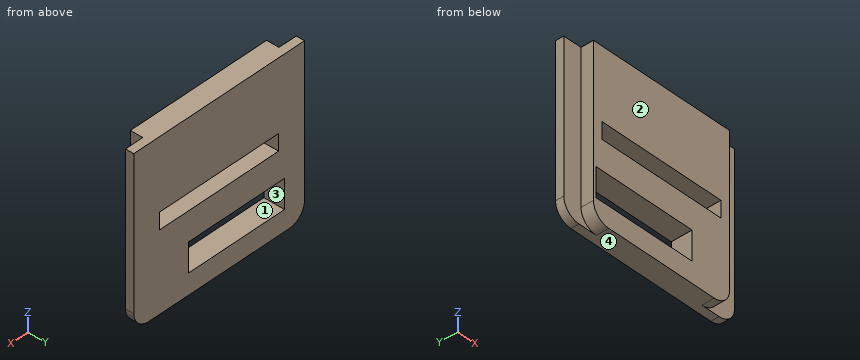
from build123d import *

# Parameters (mm, degrees)
F1_DEPTH = 1
F3_DEPTH = 1.5
F5_W     = 12.5
F5_H     = 3.5
F5_W_2   = 15.5
F5_H_2   = 2
F6_DEPTH = 2.5


with BuildPart() as f1:
    # F0 (on Front) → F1 (new body)
    with BuildSketch(Plane.XZ):
        with BuildLine():
            ThreePointArc((0, 2), (0.585786, 0.585786), (2, 0))
            Line((2, 0), (20.25, 0))
            ThreePointArc((20.25, 0), (21.664214, 0.585786), (22.25, 2))
            Line((22.25, 2), (22.25, 20))
            Line((22.25, 20), (0, 20))
            Line((0, 20), (0, 2))
        make_face()
    extrude(amount=F1_DEPTH)


with BuildPart() as f3:
    # F2 (on face) → F3 (new body)
    with BuildSketch(Plane.XZ.offset(1)):
        with BuildLine():
            Line((20, 20), (2.25, 20))
            Line((2.25, 20), (2.25, 2))
            ThreePointArc((2.25, 2), (2.835786, 0.585786), (4.25, 0))
            Line((4.25, 0), (18, 0))
            ThreePointArc((18, 0), (19.414214, 0.585786), (20, 2))
            Line((20, 2), (20, 20))
        make_face()
    extrude(amount=F3_DEPTH)


with BuildPart() as f1_1:
    add(f1.part)

    # F4: union F3
    add(f3.part)

    # F5 (on face) → F6 (cut, through all)
    with BuildSketch(Plane(origin=(0, 0, 0), x_dir=(-1, 0, 0), z_dir=(0, 1, 0))):
        with Locations((-8.85, 4.25)):
            Rectangle(F5_W, F5_H)
        with Locations((-11.125, 10.5)):
            Rectangle(F5_W_2, F5_H_2)
    extrude(amount=-F6_DEPTH, mode=Mode.SUBTRACT)


solid = f1_1.part
Could you check a few things on this model? Use its own coordinates, in mm. Face numbers are marked on the shaded views. A direction names the side the tool comes from. Give positions to 0.01 mm unless a question says otherwise; leave off trailing zeros. Order: outer loops, then holes, each group sorted by start corner. A loop starts at its lowest first (then second) coordinate and runs counter-clockwise, first axis right, second up. Notation, with made-up numbers: (-21, 78.5) - (28, 78.5) arc R32 ccw to (28, 111.5) - close; hole circle Ø11 at (-38, 12). An arc over 180 degrees is marked (long way). Return JSON: item names as keys, results as strings. Group by question number.
Q1. Suppose I cut it at B-B, the plane y = -0.5. Please give me the cut outline in (x, z) (3 decimals).
Q2. Which directions (+Z, -Z, +X, -X, +Y, -Y) give clear straight access to the entire face, cutting with the end or side of a thin tool? Please do the marked faces 3 and 4.
Q3. Suppose I cut it at A-A, the plane x = 10.5. Please give me the cut outline in (y, z).
Q4. Suppose I cut it at C-C, the plane z = 10.5. Please give me the cut outline in (x, y) (3 decimals), and give its area (3 significant figures).
Q5. Suppose I cut it at D-D, the plane z = 17.5. Please give me the cut outline in (x, y).
Q6. Thinking about a two-plate mould opening in X: for the marked faces 1 and 2, which applies, pulls with the +X half, pulls with the -X half, needs draft (parallel to the pull), parting line crosses it, or undercut?
Q7. Will these pins go through, and if not, where does the flat tip stop? pin 1 Ø10 at (x, z) = (15.5, 13.5) entering from +Y; pin 2 Ø1.2 at (y, z) = (-2, 8.5) entering from +X.
Q8. Please list where these lines run through material, in increasing order: line 1 along Z through (x, y) = (8.25, -1.4); line 2 along Z through (x, y) = (16.5, -1.2); line 3 along X through (y, z) = (-0.65, 3). Write a range as [from, to].
Resolved:
{
 "1": {"outline": "(0, 2) arc R2 ccw to (2, 0) - (20.25, 0) arc R2 ccw to (22.25, 2) - (22.25, 20) - (0, 20) - close; hole (2.6, 2.5) - (15.1, 2.5) - (15.1, 6) - (2.6, 6) - close; hole (3.375, 9.5) - (18.875, 9.5) - (18.875, 11.5) - (3.375, 11.5) - close"},
 "2": {"face 3": "+Y, -Y", "face 4": "-Z, +X, -X, +Y, -Y"},
 "3": {"outline": "(-2.5, 0) - (0, 0) - (0, 2.5) - (-2.5, 2.5) - close; (-2.5, 6) - (0, 6) - (0, 9.5) - (-2.5, 9.5) - close; (-2.5, 11.5) - (0, 11.5) - (0, 20) - (-2.5, 20) - close"},
 "4": {"outline": "(0, -1) - (2.25, -1) - (2.25, -2.5) - (3.375, -2.5) - (3.375, 0) - (0, 0) - close; (18.875, -2.5) - (20, -2.5) - (20, -1) - (22.25, -1) - (22.25, 0) - (18.875, 0) - close", "area": "10.1 mm2"},
 "5": {"outline": "(0, -1) - (2.25, -1) - (2.25, -2.5) - (20, -2.5) - (20, -1) - (22.25, -1) - (22.25, 0) - (0, 0) - close"},
 "6": {"face 1": "undercut", "face 2": "needs draft"},
 "7": {"pin 1": "stops at y = 0", "pin 2": "stops at x = 20"},
 "8": {"line 1": "z = [0, 2.5], [6, 9.5], [11.5, 20]", "line 2": "z = [0, 9.5], [11.5, 20]", "line 3": "x = [0, 2.6], [15.1, 22.25]"}
}
